Read the model definition and answer for the solid it produces. Units are mm, in the model's axes. A direction names the side the tool comes from. Round coordinates to 2 decimals unless told otherwise and drop trailing zeros. Order: outer loops, then holes, each group sorted by start corner. A loop starts at its lowest first (then second) coordinate and runs counter-clockwise, first axis right, second up. Notation, with made-up numbers: M -27,32.5 L -21,32.5 A14 cw -21,39.5 Z; hole C 10,-4.5 d6. An arc over 180 degrees is marked long. Answer as CSV lines item,"result".
```python
from build123d import *

# Parameters (mm, degrees)
F0_W     = 40
F0_H     = 20
F1_DEPTH = 1
F0_W_2   = 4
F0_W_3   = 69
F2_DEPTH = 2
F4_DEPTH = 2
F5_R     = 0.5


with BuildPart() as f1:
    # F0 (on Top) → F1 (new body)
    with BuildSketch(Plane.XY):
        with Locations((0.652443, -3.960167)):
            Rectangle(F0_W, F0_H)
    extrude(amount=F1_DEPTH)

    # F0 (on Top) → F2 (join)
    with BuildSketch(Plane.XY):
        with Locations((22.652443, -3.960167)):
            Rectangle(F0_W_2, F0_H)
        with Locations((-21.347557, -3.960167)):
            Rectangle(F0_W_2, F0_H)
        with Locations((59.152443, -3.960167)):
            Rectangle(F0_W_3, F0_H)
    extrude(amount=F2_DEPTH)

    # F3 (on face) → F4 (join)
    with BuildSketch(Plane.XY.offset(2)):
        Polygon((20.652443, 6.039833), (20.652443, -13.960167), (23.152443, -13.960167), (23.152443, -5.210167), (91.152443, -5.210167), (91.152443, -13.960167), (93.652443, -13.960167), (93.652443, 6.039833), (91.152443, 6.039833), (91.152443, -2.710167), (23.152443, -2.710167), (23.152443, 6.039833), align=None)
    extrude(amount=F4_DEPTH)

    # F5
    f5_edges = [f1.edges().sort_by_distance(p)[0] for p in [
        (21.902443, 6.039833, 4),
        (20.652443, -3.960167, 4),
        (21.902443, -13.960167, 4),
        (23.152443, -9.585167, 4),
        (57.152443, -5.210167, 4),
        (91.152443, -9.585167, 4),
        (92.402443, -13.960167, 4),
        (93.652443, -3.960167, 4),
        (92.402443, 6.039833, 4),
        (91.152443, 1.664833, 4),
        (57.152443, -2.710167, 4),
        (23.152443, 1.664833, 4),
    ]]
    fillet(f5_edges, radius=F5_R)


solid = f1.part
```
Item 1: A cutting plane is placed at C-C, the plane y = -0.75. Determine the outline of the cut face in (x, z), and give its area (3 significant figures).
Ans:
outline,"M -23.35,0 L 93.65,0 L 93.65,3.5 A0.5 ccw 93.15,4 L 91.65,4 A0.5 ccw 91.15,3.5 L 91.15,2 L 23.15,2 L 23.15,3.5 A0.5 ccw 22.65,4 L 21.15,4 A0.5 ccw 20.65,3.5 L 20.65,1 L -19.35,1 L -19.35,2 L -23.35,2 Z"
area,"204 mm2"
Item 2: A cutting plane is placed at B-B, the plane x = 41. Determine the outline of the cut face in (y, z).
Ans:
outline,"M -13.96,0 L 6.04,0 L 6.04,2 L -2.71,2 L -2.71,3.5 A0.5 ccw -3.21,4 L -4.71,4 A0.5 ccw -5.21,3.5 L -5.21,2 L -13.96,2 Z"
Item 3: A tool of negligible diameter and unlimited length cuts with its end or side. For faces 4 (the face through (57, 2, 2)), 5 (the face through (-21, -4, 2)), 6 (the face through (0, -4, 1)), 7 (the face through (57, -10, 2)), from which of +Z, -Z, +X, -X, +Y, -Y can it reach the whole face along a straight path? Write none if from no direction.
Ans:
face 4,"+Z, +Y"
face 5,"+Z, -X, +Y, -Y"
face 6,"+Z, +Y, -Y"
face 7,"+Z, -Y"
Item 4: Find the intervals of material crossed by probe 1 along X at (y, z) = (3.5, 1.75); probe 2 along X at (y, z) = (-5.25, 2.8); probe 3 along Z at (x, y) = (-2, 0.75), in increasing order. Write a range as [from, to].
Ans:
probe 1,"[-23.35, -19.35], [20.65, 93.65]"
probe 2,"[20.65, 23.15], [91.15, 93.65]"
probe 3,"[0, 1]"
Item 5: A cutting plane is placed at A-A, the plane z = 2.7. Determine the outline of the cut face in (x, y), and give its area (3 significant figures).
Ans:
outline,"M 20.65,-13.96 L 23.15,-13.96 L 23.15,-5.21 L 91.15,-5.21 L 91.15,-13.96 L 93.65,-13.96 L 93.65,6.04 L 91.15,6.04 L 91.15,-2.71 L 23.15,-2.71 L 23.15,6.04 L 20.65,6.04 Z"
area,"270 mm2"
Item 6: A cutting plane is placed at D-D, the plane x = 17.5. Determine the outline of the cut face in (y, z).
Ans:
outline,"M -13.96,0 L 6.04,0 L 6.04,1 L -13.96,1 Z"
Item 7: Determine the mould class of faces 1 (the face through (34, -13.96, 1)), 2 (the face through (-23.348, -4, 1)), 3 (the face through (20.652, -4, 2)) for opening direction X: +X half, -X half, draft (parallel to the pull), parting line (faces both ways), or undercut.
Ans:
face 1,"draft"
face 2,"-X half"
face 3,"undercut"
Item 8: Flat-ended cylindrical pins translate along their axes: pin 1 (7 mm diameter, centred on x = 41.5, y = 2, fed in from +Z); pin 2 (1.6 mm diameter, centred on x = 63.5, z = 3, fed in from +Y); pin 3 (1.2 mm diameter, centred on y = -8.5, z = 3, fed in from -X). Find the tip coordinate at first contact, or state that the pin passes through.
Ans:
pin 1,"z = 2"
pin 2,"y = -2.71"
pin 3,"x = 20.65"
